```python
from build123d import *

# Parameters (mm, degrees)
SKETCH1_W                 = 36
SKETCH1_H                 = 17
BOSS_EXTRUDE1_DEPTH       = 1.5
SKETCH2_W                 = 10
SKETCH2_H                 = 10
BOSS_EXTRUDE2_DEPTH       = 4
SKETCH3_W                 = 10
SKETCH3_H                 = 10
BOSS_EXTRUDE3_DEPTH       = 5
SKETCH4_R                 = 1
CUT_EXTRUDE1_DEPTH        = 5
LPATTERN1_COUNT           = 2
LPATTERN1_PITCH           = 7
LPATTERN2_COUNT           = 2
LPATTERN2_PITCH           = 30
LPATTERN2_COPY_1_SKETCH_R = 1
LPATTERN2_COPY_1_DEPTH    = 5


with BuildPart() as part:
    # Sketch1 → Boss-Extrude1 (new body)
    with BuildSketch(Plane(origin=(0, 0, 0), x_dir=(1, 0, 0), z_dir=(0, 1, 0))):
        with Locations((18, -8.5)):
            Rectangle(SKETCH1_W, SKETCH1_H)
    extrude(amount=BOSS_EXTRUDE1_DEPTH)

    # Sketch2 → Boss-Extrude2 (add)
    with BuildSketch(Plane(origin=(0, 1.5, 0), x_dir=(1, 0, 0), z_dir=(0, 1, 0))):
        with Locations((23, -5)):
            Rectangle(SKETCH2_W, SKETCH2_H)
    extrude(amount=BOSS_EXTRUDE2_DEPTH)

    # Sketch3 → Boss-Extrude3 (add)
    with BuildSketch(Plane(origin=(0, 1.5, 0), x_dir=(1, 0, 0), z_dir=(0, 1, 0))):
        with Locations((12, -12)):
            Rectangle(SKETCH3_W, SKETCH3_H)
    extrude(amount=BOSS_EXTRUDE3_DEPTH)

    # Sketch4 → Cut-Extrude1 (cut)
    with BuildSketch(Plane(origin=(0, 1.5, 0), x_dir=(1, 0, 0), z_dir=(0, 1, 0))):
        with Locations(Location((3, -5, 0), (0, 0, 270))):
            Circle(SKETCH4_R)
    cut_extrude1 = extrude(amount=-CUT_EXTRUDE1_DEPTH, mode=Mode.SUBTRACT)

    # LPattern1: Cut-Extrude1 ×2
    with Locations(*[(0, 0, i * LPATTERN1_PITCH) for i in range(1, LPATTERN1_COUNT)]):
        add(cut_extrude1, mode=Mode.SUBTRACT)

    # LPattern2: Cut-Extrude1 ×2
    with Locations(*[(i * LPATTERN2_PITCH, 0, 0) for i in range(1, LPATTERN2_COUNT)]):
        add(cut_extrude1, mode=Mode.SUBTRACT)

    # LPattern2 copy 1 sketch → LPattern2 copy 1 (cut)
    with BuildSketch(Plane(origin=(30, 1.5, 7), x_dir=(1, 0, 0), z_dir=(0, 1, 0))):
        with Locations(Location((3, -5, 0), (0, 0, 270))):
            Circle(LPATTERN2_COPY_1_SKETCH_R)
    extrude(amount=-LPATTERN2_COPY_1_DEPTH, mode=Mode.SUBTRACT)


solid = part.part
```
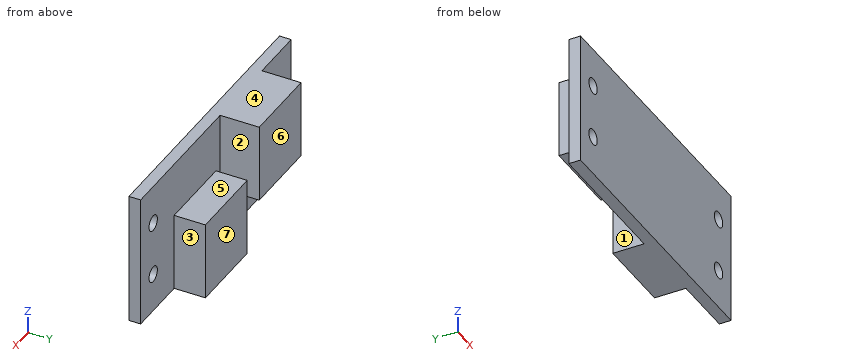
Read the model definition and answer for the solid it produces. Units are mm, in the model's axes. Face numbers are marked on the shaded views. A direction names the side the tool comes from. Coordinates: 2 decimals unless noted, no trailing zeros. Loops run counter-clockwise (first coordinate to the right, second up) from the corner with the lowest first, then second, coordinate; pieces in that order, holes last.
(1) The mould has two halves that part along X. Classify the marked faces 1, 2, 3 and 4: released by +X, released by -X, zero draft, split by the parting line, or undercut.
Solution:
face 1: undercut
face 2: undercut
face 3: released by +X
face 4: zero draft
(2) Flat-ended cylindrical pins translate along their axes: pin 1 Ø1.5 at (y, z) = (4, 12) entering from -X; pin 2 Ø1.5 at (y, z) = (1, 12.5) entering from -X; pin 3 Ø8 at (x, z) = (23.5, 2.5) entering from +Y; pin 4 Ø3 at (x, z) = (33, 5) entering from +Y. Find the tip coordinate at first contact, or state that the pin passes through.
Solution:
pin 1: stops at x = 7
pin 2: stops at x = 0
pin 3: stops at y = 5.5
pin 4: stops at y = 1.5
(3) Consider line 1 along X through (y, z) = (0.85, 5); line 2 along X through (y, z) = (4.25, 9.5); line 3 along Y through (x, z) = (21.5, 1.5). Determine where each line is inside the solid, lowest interval first.
Solution:
line 1: x = 0 to 2, 4 to 32, 34 to 36
line 2: x = 7 to 17, 18 to 28
line 3: y = 0 to 5.5
(4) A tool of negligible diameter and unlimited length cuts with its end or side. For the marked faces 5, 6 and 7, from which of +Z, -Z, +X, -X, +Y, -Y can it reach the whole face along a straight path? Write none if from no direction.
Solution:
face 5: +Z, +X, +Y
face 6: +Z, -Z, +X, -X, +Y
face 7: +Z, -Z, +X, +Y
(5) The part is cut by section B-B (z = 12). Determine the outline of the cut face in (x, y).
Solution:
outline: (0, 0) - (2, 0) - (2, 1.5) - (0, 1.5) - close; (4, 0) - (32, 0) - (32, 1.5) - (17, 1.5) - (17, 6.5) - (7, 6.5) - (7, 1.5) - (4, 1.5) - close; (34, 0) - (36, 0) - (36, 1.5) - (34, 1.5) - close
(6) The part is cut by section A-A (x = 3). Determine the outline of the cut face in (y, z), and give its area (3 significant figures).
Solution:
outline: (0, 0) - (1.5, 0) - (1.5, 4) - (0, 4) - close; (0, 6) - (1.5, 6) - (1.5, 11) - (0, 11) - close; (0, 13) - (1.5, 13) - (1.5, 17) - (0, 17) - close
area: 19.5 mm2
(7) The part is cut by section C-C (y = 2.5). Determine the outline of the cut face in (x, z).
Solution:
outline: (7, 7) - (17, 7) - (17, 17) - (7, 17) - close; (18, 0) - (28, 0) - (28, 10) - (18, 10) - close
(8) The part is cut by section D-D (z = 3). Determine the outline of the cut face in (x, y), and give its area (3 significant figures).
Solution:
outline: (0, 0) - (36, 0) - (36, 1.5) - (28, 1.5) - (28, 5.5) - (18, 5.5) - (18, 1.5) - (0, 1.5) - close
area: 94.0 mm2
